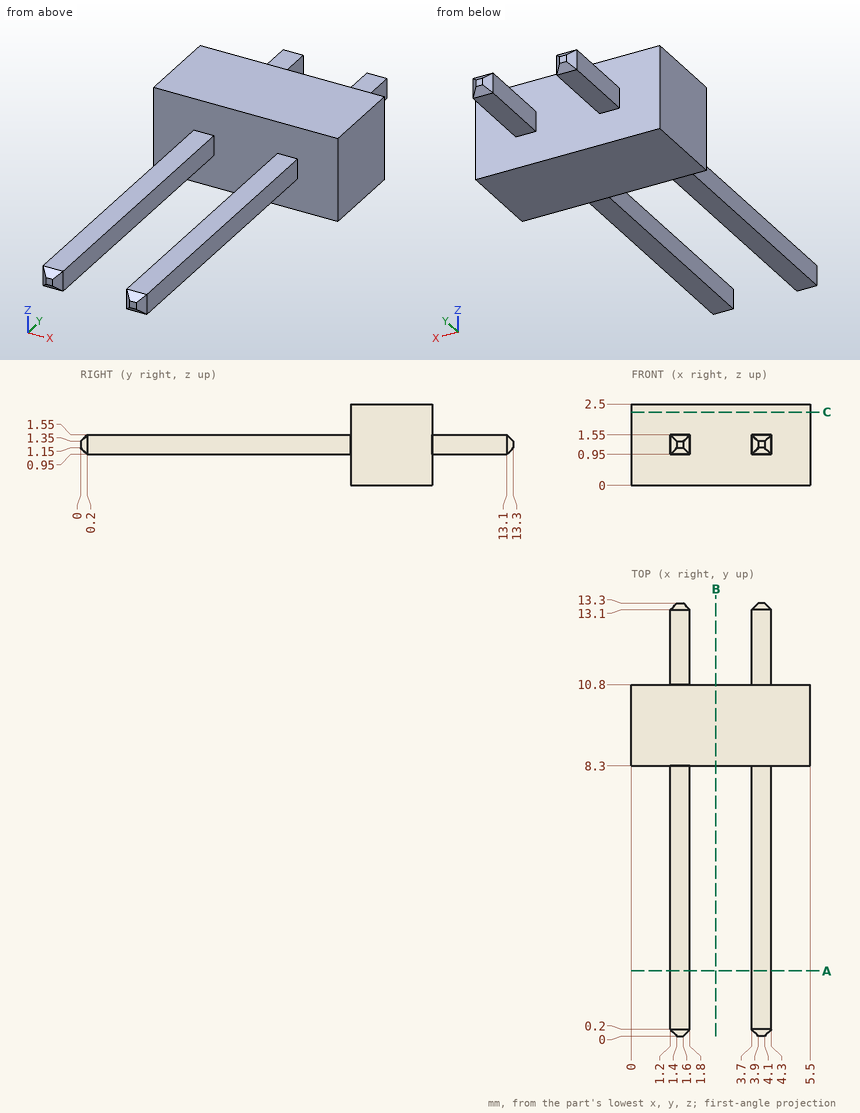
Geometry: see drawing. Coordinates: mm, zero at the bounding-box minimum. Give positions to 0.01 mm unless a question says otherwise; leave off trailing zeros. Order: outer loops, then holes, each group sorted by start corner. A loop starts at its lowest first (then second) coordinate and runs counter-clockwise, first axis right, second up. Notation, with made-up numbers: (37.5, 86.5) -> (60.5, 86.5) arc R25 cw to (60.5, 99.5) -> close; hole circle Ø3 at (-24, 53.5). An arc over 180 degrees is marked (long way). Write each question's results on one line, items separated by ' | '.
1) Cut plane A-A (y = 2). Output: boundary loops of the cut face in (x, z).
Geometry says:
outline: (1.2, 0.95) -> (1.8, 0.95) -> (1.8, 1.55) -> (1.2, 1.55) -> close; (3.7, 0.95) -> (4.3, 0.95) -> (4.3, 1.55) -> (3.7, 1.55) -> close
2) First-contact query: pin 1 Ø0.7 at (x, y) = (1.5, 12.5) entering from -Z; pin 2 Ø1.2 at (x, z) = (3, 1.5) entering from -Y; pin 3 Ø0.7 at (y, z) = (12.5, 1) entering from -X. Flat tips, straight axial feed; report the tip coordinate or a pass-through.
Geometry says:
pin 1: stops at z = 0.95 | pin 2: stops at y = 8.3 | pin 3: stops at x = 1.2
3) Cut plane C-C (z = 2.25). Output: boundary loops of the cut face in (x, y), and give its area (4 significant figures).
Geometry says:
outline: (0, 8.3) -> (5.5, 8.3) -> (5.5, 10.8) -> (0, 10.8) -> close | area: 13.75 mm²
4) Cut plane B-B (x = 2.6). Output: boundary loops of the cut face in (y, z).
Geometry says:
outline: (8.3, 0) -> (10.8, 0) -> (10.8, 2.5) -> (8.3, 2.5) -> close
5) Line query: line 1 along X through (y, z) = (7, 1.35); line 2 along Z through (x, y) = (4.2, 12); line 3 along Y through (x, z) = (1.75, 0.2). Output: solid intervals per line, ascending.
Geometry says:
line 1: x = 1.2 to 1.8, 3.7 to 4.3 | line 2: z = 0.95 to 1.55 | line 3: y = 8.3 to 10.8
